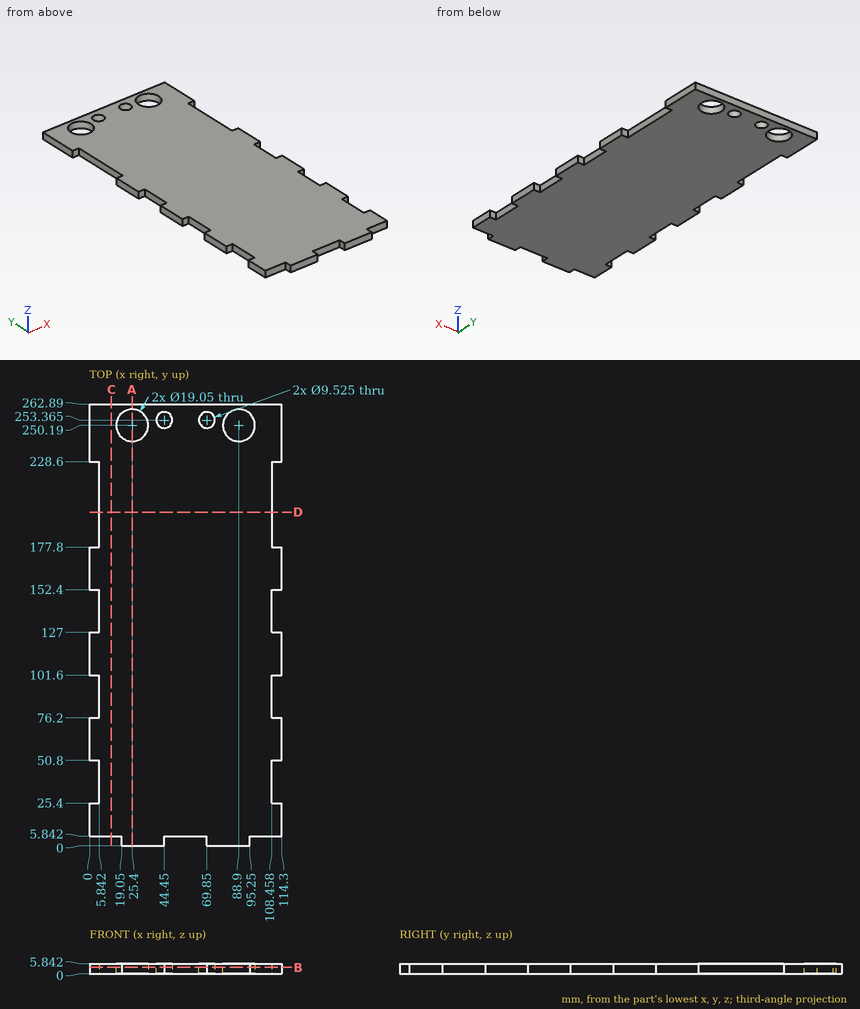
Input: dimensioned drawing with shaded views. Units: mm. Origin: part minimum x, y, z. Round coordinates to 2 decimals unless told otherwise and drop trailing zeros. Loops run counter-clockwise (first coordinate to the right, second up) from the corner with the lowest first, then second, coordinate; pieces in that order, holes last. Notation, with made-up numbers: (70, 10) -> (81, 10) arc R20 ccw to (81, 36) -> close; hole circle Ø3 at (73, 73). An arc over 180 degrees is marked (long way). One line per item, written item: value.
(1) Pin query (flat end, axial travel): pin 1 (7.5 mm diameter, centred on x = 69.85, y = 253.365, fed in from +Z); pin 2 (3 mm diameter, centred on x = 56, z = 3, fed in from -Y); pin 3 (1.8 mm diameter, centred on y = 33.5, z = 3.5, fed in from -X); pin 4 (1.5 mm diameter, centred on y = 81.5, z = 2.5, fed in from +X). Return the tip coordinate at first contact, or that it passes through.
Geometry check:
pin 1: through
pin 2: y = 5.84
pin 3: x = 5.84
pin 4: x = 108.46
(2) Section C-C (x = 13). Return the cut outline in (y, z), plus the area to 3 significant figures.
Geometry check:
outline: (5.84, 0) -> (262.89, 0) -> (262.89, 5.84) -> (5.84, 5.84) -> close
area: 1,500 mm2
(3) Material intervals for line 1 (Y direction, x = 108.5, z = 2.8); line 2 (Y direction, x = 25.4, z = 1.4) (3 decimals); line 3 (X direction, y = 248, z = 1), sorted ascending. Write a range as [from, to].
Geometry check:
line 1: [5.84, 25.4], [50.8, 76.2], [101.6, 127], [152.4, 177.8], [228.6, 262.89]
line 2: [0, 240.665], [259.715, 262.89]
line 3: [0, 16.13], [34.67, 79.63], [98.17, 114.3]
(4) Section B-B (z = 3.75). Give the number of separate pieces and of enclosed holes in the cut face, plus the area to 3 significant figures.
Geometry check:
separate pieces: 1
enclosed holes: 4
area: 27,500 mm2
(5) Section D-D (y = 198.5). Return the cut outline in (x, z), plus the area to 3 significant figures.
Geometry check:
outline: (5.84, 0) -> (108.46, 0) -> (108.46, 5.84) -> (5.84, 5.84) -> close
area: 599 mm2
(6) Section A-A (x = 25.4). Return the cut outline in (y, z) (3 decimals), plus the area to 3 significant figures.
Geometry check:
outline: (0, 0) -> (240.665, 0) -> (240.665, 5.842) -> (0, 5.842) -> close; (259.715, 0) -> (262.89, 0) -> (262.89, 5.842) -> (259.715, 5.842) -> close
area: 1,420 mm2
